Could you check a few things on this model? Use its own coordinates, in mm. A direction names the side the tool comes from. Give positions to 0.01 mm unless a question says otherwise; leave off trailing zeros. Loops run counter-clockwise (first coordinate to the right, second up) from the corner with the lowest first, then second, coordinate; pieces in that order, holes last. Notation, with made-up numbers: (19, 81) -> (60, 81) arc R30 ccw to (60, 110) -> close; hole circle Ø1 at (3, 20.5). An arc over 180 degrees is marked (long way). Put each result on its own line as item: value.
```python
from build123d import *

# Parameters (mm, degrees)
PAD_DEPTH    = 8
FILLET_R     = 0.5
SKETCH002_W  = 5
SKETCH002_H  = 16
PAD002_DEPTH = 2
SKETCH001_W  = 10
SKETCH001_H  = 16
SKETCH001_R  = 2.25
PAD001_DEPTH = 6
CHAMFER_SIZE = 2


with BuildPart() as obj1:
    # Sketch → Pad (new body)
    with BuildSketch(Plane.XY):
        Polygon((0, 0), (5, 0), (5, -16), (0, -16), (0, -10), (3, -11), (3, -5), (0, -6), align=None)
        Polygon((15, 0), (15, -16), (17, -16), (17, -9.5), (20, -10.5), (20, -5.5), (17, -6.5), (17, 0), align=None)
    extrude(amount=PAD_DEPTH)

    # Fillet
    fillet_edges = [obj1.edges().sort_by_distance(p)[0] for p in [
        (0, -6, 4),
        (0, -10, 4),
        (20, -5.5, 4),
        (20, -10.5, 4),
    ]]
    fillet(fillet_edges, radius=FILLET_R)


with BuildPart() as pad002:
    # Sketch002 → Pad002 (new body)
    with BuildSketch(Plane.XY.offset(8)):
        with Locations((2.5, -8)):
            Rectangle(SKETCH002_W, SKETCH002_H)
        with Locations((17.5, -8)):
            Rectangle(SKETCH002_W, SKETCH002_H)
    extrude(amount=PAD002_DEPTH)


with BuildPart() as fusion:
    # Sketch001 → Pad001 (new body)
    with BuildSketch(Plane.XY):
        with Locations((10, -8)):
            Rectangle(SKETCH001_W, SKETCH001_H)
        with Locations((10, -8)):
            Circle(SKETCH001_R, mode=Mode.SUBTRACT)
    extrude(amount=PAD001_DEPTH)

    # Chamfer
    chamfer_edges = [fusion.edges().sort_by_distance(p)[0] for p in [
        (7.75, -8, 6),
    ]]
    chamfer(chamfer_edges, length=CHAMFER_SIZE)

    # Fusion: union obj1, Pad002
    add(obj1.part)
    add(pad002.part)


solid = fusion.part
```
1. If we section it at D-D (z = 4.75): List the corners of the cut face in (x, y) for me, then the cut area to 3 significant figures.
Recorded:
outline: (0, -16) -> (17, -16) -> (17, -9.5) -> (19.34, -10.28) arc R0.5 ccw to (20, -9.81) -> (20, -6.19) arc R0.5 ccw to (19.34, -5.72) -> (17, -6.5) -> (17, 0) -> (0, 0) -> (0, -5.31) arc R0.5 ccw to (0.66, -5.78) -> (3, -5) -> (3, -11) -> (0.66, -10.22) arc R0.5 ccw to (0, -10.69) -> close; hole circle Ø6 at (10, -8)
area: 240 mm^2
2. If we section it at B-B (z = 9): List the corners of the cut face in (x, y) for me, then the cut area to 3 significant figures.
Recorded:
outline: (0, -16) -> (5, -16) -> (5, 0) -> (0, 0) -> close; (15, -16) -> (20, -16) -> (20, 0) -> (15, 0) -> close
area: 160 mm^2
3. If we section it at A-A (x = 10): List the corners of the cut face in (y, z) for me, then the cut area to 3 significant figures.
Recorded:
outline: (-16, 0) -> (-10.25, 0) -> (-10.25, 4) -> (-12.25, 6) -> (-16, 6) -> close; (-5.75, 0) -> (0, 0) -> (0, 6) -> (-3.75, 6) -> (-5.75, 4) -> close
area: 65.0 mm^2
4. I'm going to push flat-ended pins straight in: pin 1 (4 mm diameter, centred on x = 10, y = -8, fed in from +Z); pin 2 (4 mm diameter, centred on x = 7.5, y = -5, fed in from +Z); pin 3 (1.5 mm diameter, centred on x = 19, y = -14, fed in from -Z). Where does each tip first touch, or does it pass through?
Recorded:
pin 1: passes through
pin 2: stops at z = 6
pin 3: stops at z = 8
5. If we section it at C-C (y = -8): List the corners of the cut face in (x, z) for me, then the cut area to 3 significant figures.
Recorded:
outline: (0, 8) -> (3, 8) -> (3, 0) -> (7.75, 0) -> (7.75, 4) -> (5.75, 6) -> (5, 6) -> (5, 10) -> (0, 10) -> close; (12.25, 0) -> (20, 0) -> (20, 10) -> (15, 10) -> (15, 6) -> (14.25, 6) -> (12.25, 4) -> close
area: 105 mm^2
6. Thinking about a two-plate mould opening in X: for faces 1 (the face through (0, -8.1, 8.3)), 2 (the face through (5, -8, 8)), 3 (the face through (8, -10, 0)), which applies, pulls with the +X half, pulls with the -X half, needs draft (parallel to the pull), parting line crosses it, or undercut?
Recorded:
face 1: pulls with the -X half
face 2: undercut
face 3: needs draft
7. For faces 4 (the face through (3, -8, 4)), 5 (the face through (18.2, -9.9, 3.9)), 6 (the face through (15, -8, 8)), which set-ups out of +Z, -Z, +X, -X, +Y, -Y let a thin tool reach every point of the face, with its end or its side?
Recorded:
face 4: -Z
face 5: -Z, -Y
face 6: +Z, +Y, -Y
8. I need wall thicknesses on line 1 (Y direction, x = 10, z = 2); line 2 (X direction, y = -0.75, z = 9.5); line 3 (X direction, y = -8, z = 7). Which ranges of each line are inside material? Lowest first, please.
Recorded:
line 1: y = -16 to -10.25, -5.75 to 0
line 2: x = 0 to 5, 15 to 20
line 3: x = 3 to 5, 15 to 20
